from build123d import *

# Parameters (mm, degrees)
ESBO_O1_W                = 103
ESBO_O1_H                = 34
RESSALTO_EXTRUS_O1_DEPTH = 24
CORTE_EXTRUS_O1_DEPTH    = 0.5
FILETE1_R                = 2


with BuildPart() as part:
    # Esboço1 → Ressalto-extrusão1 (new body)
    with BuildSketch(Plane.XY):
        Rectangle(ESBO_O1_W, ESBO_O1_H)
    extrude(amount=RESSALTO_EXTRUS_O1_DEPTH)

    # Esboço2 → Corte-extrusão1 (cut)
    with BuildSketch(Plane(origin=(51.5, 0, 0), x_dir=(0, 0, -1), z_dir=(1, 0, 0))):
        with BuildLine():
            Line((-4.5, 6), (-4.5, -6))
            ThreePointArc((-4.5, -6), (-12, -13.5), (-19.5, -6))
            Line((-19.5, -6), (-19.5, 6))
            ThreePointArc((-19.5, 6), (-12, 13.5), (-4.5, 6))
        make_face()
    corte_extrus_o1 = extrude(amount=-CORTE_EXTRUS_O1_DEPTH, mode=Mode.SUBTRACT)

    # Espelhar1: Corte-extrusão1 across plane
    add(corte_extrus_o1.mirror(Plane(origin=(0, 0, 0), x_dir=(0, 0, 1), z_dir=(1, 0, 0))), mode=Mode.SUBTRACT)

    # Filete1
    filete1_edges = [part.edges().sort_by_distance(p)[0] for p in [
        (-51.5, 0, 24),
        (0, -17, 24),
        (51.5, 0, 24),
        (0, -17, 0),
        (-51.5, 0, 0),
        (0, 17, 0),
        (51.5, 0, 0),
        (0, 17, 24),
        (51.5, -17, 12),
        (-51.5, -17, 12),
        (-51.5, 17, 12),
        (51.5, 17, 12),
    ]]
    fillet(filete1_edges, radius=FILETE1_R)


solid = part.part
Model file for the job. Use its own axes, mm. A direction names the side the tool comes from. Give positions to 0.01 mm unless a question says otherwise; leave off trailing zeros.
1) Wall check: line 1 (X direction, y = 6, z = 17); line 2 (Y direction, x = -25.5, z = 1.75); line 3 (X direction, y = 13.5, z = 22.5). Give the ranges that are in metal, low to high.
2) Pull direction Z, two halves, no side cores. Call faces 1 (the cylindrical face through (0.69, -16.43, 0.6)), 2 (the flat face through (-51.5, 0, 3)), 3 (the cylindrical face through (-51.25, 13.5, 12.16)): +Z half, -Z half, draft (parallel to the pull), parting line (faces both ways), or undercut.
3) Tool access for faces 4 (the cylindrical face through (51.25, 13.5, 12.16)), 5 (the flat face through (-1, 0, 24)), 6 (the flat face through (-51, 0, 12)): list every direction of +Z, -Z, +X, -X, +Y, -Y with a clear straight run to the whole face (end or side of a thin tool).
4) Flat gauge pins, fed straight in: pin 1 Ø2 at (y, z) = (3.5, 6) entering from -X; pin 2 Ø0.6 at (x, y) = (51.5, -2.5) entering from +Z. Where does each tip first touch, or does it go through?
Answer block:
1. line 1: x = -51 to 51
1. line 2: y = -16.98 to 16.98
1. line 3: x = -51.44 to 51.44
2. face 1: -Z half
2. face 2: draft
2. face 3: undercut
3. face 4: +X
3. face 5: +Z, +X, -X, +Y, -Y
3. face 6: -X
4. pin 1: stops at x = -51
4. pin 2: stops at z = 23.05
